```python
from build123d import *

# Parameters (mm, degrees)
F9_DEPTH      = 3.175
F9_DEPTH_BACK = 6.35
F7_R          = 3.175
F10_DEPTH     = 3.176
F3_R          = 13.0054161967
F4_R          = 1.5875
F11_DEPTH     = 6.351


# Not quite as in the source:
# - a variable given as a bare number and used for a length is read in inches; the dataset says mm whatever the document's units were


with BuildPart() as f9:
    # F1 (on Front) → F9 (new body, two sides)
    with BuildSketch(Plane.XZ) as f9_sk:
        with BuildLine():
            Line((0, 50.8), (0, 0))
            Line((0, 0), (50.8, 0))
            Line((50.8, 0), (50.8, 25.4))
            ThreePointArc((50.8, 25.4), (32.8394877579, 32.8394877579), (25.4, 50.8))
            Line((25.4, 50.8), (0, 50.8))
        make_face()
    extrude(amount=F9_DEPTH)
    extrude(f9_sk.sketch, amount=-F9_DEPTH_BACK)

    # F8 (on Front) + F7 (on Front) → F10 (cut, through all)
    with BuildSketch(Plane.XZ):
        with BuildLine():
            Line((22.8825640303, 25.1276280605), (21.4592504682, 23.7043144985))
            Line((21.4592504682, 23.7043144985), (23.7043144985, 21.4592504682))
            Line((23.7043144985, 21.4592504682), (25.1276280605, 22.8825640303))
            ThreePointArc((25.1276280605, 22.8825640303), (25.1276280605, 25.1276280605), (22.8825640303, 25.1276280605))
        make_face()
    with BuildSketch(Plane.XZ):
        with Locations((20.6375, 20.6375)):
            Circle(F7_R)
    extrude(amount=F10_DEPTH, mode=Mode.SUBTRACT)

    # F3 (on Front) + F4 (on Front) + F6 (on face) → F11 (cut, through all)
    with BuildSketch(Plane.XZ):
        with Locations((20.6375, 20.6375)):
            Circle(F3_R)
    with BuildSketch(Plane.XZ):
        with Locations((37.4589580984, 20.6375)):
            Circle(F4_R)
        with Locations((20.6375, 37.4589580984)):
            Circle(F4_R)
        with Locations((5.159375, 5.159375)):
            Circle(F4_R)
    with BuildSketch(Plane.XZ):
        Polygon((17.0707799442, 8.1307274949), (13.0054161967, 0), (28.2695838033, 0), (24.7028637475, 8.1307274949), align=None)
        Polygon((8.1307274949, 24.7028637475), (0, 28.2695838033), (0, 13.0054161967), (8.1307274949, 17.0707799442), align=None)
    extrude(amount=-F11_DEPTH, mode=Mode.SUBTRACT)


solid = f9.part
```
Could you check a few things on this model? Use its own coordinates, in mm. A direction names the side the tool comes from. Coordinates: 2 decimals unless noted, no trailing zeros. Write each loop counter-clockwise with the first axis right and the second up, starting at its lowest first coordinate (ties: lowest second). Pieces come first, ordered by that corner, then holes. Notation, with made-up numbers: (58.5, 26) -> (71.5, 26) arc R13 ccw to (71.5, 30) -> close; hole circle Ø10 at (2.25, -3.75). An arc over 180 degrees is marked (long way). Write item = value, one per line. Start each with the question number.
(1) I want a section at D-D (z = 14.5). Please give me the cut outline in (x, y) (3 decimals), plus the area to 3 significant figures.
(2) We'd pull the mould along Z, two halves only. Please class faces 4 (the face through (31, 6.35, 31)), 5 (the face through (17, 0, 17)), 6 (the face through (13, 2, 50.8)), 7 (the face through (4.01, 3.13, 15.01)): released by +Z, released by -Z, zero draft, split by the parting line, or undercut.
(3) Will these pins go through, and if not, where does the flat tip stop? pin 1 (2 mm diameter, centred on x = 23.5, y = 2.5, fed in from -Z); pin 2 (1 mm diameter, centred on x = 38, z = 20, fed in from +Y).
(4) I want a section at C-C (z = 26.5). Please give me the cut outline in (x, y) (3 decimals), plus the area to 3 significant figures.
(5) Which directions (+Z, -Z, +X, -X, +Y, -Y) give clear straight access to the entire face, cutting with the end or side of a thin tool? Please do faces 1 (the face through (4.122, 3.131, 26.461)), 2 (the face through (15.067, 3.131, 4.122)), 3 (the face through (4.82, 3.13, 3.61)).
(6) I need wall thicknesses on line 1 (Z direction, x = 20.5, y = 5.5); line 2 (Z direction, x = 5.5, y = 1.75). Which ranges of each line are inside material? Lowest first, please. Write a range as [from, to].
(7) I want a section at B-B (x = 31.5). Please give me the cut outline in (y, z) (3 decimals), plus the area to 3 significant figures.
Result set:
q1.outline = (0, -3.175) -> (50.8, -3.175) -> (50.8, 6.35) -> (32.104, 6.35) -> (32.104, 0) -> (9.171, 0) -> (9.171, 6.35) -> (2.989, 6.35) -> (2.989, 0) -> (0, 0) -> close
q1.area = 319 mm2
q2.face_4 = zero draft
q2.face_5 = undercut
q2.face_6 = released by +Z
q2.face_7 = undercut
q3.pin_1 = 8.13
q3.pin_2 = 0
q4.outline = (0, -3.175) -> (43.406, -3.175) -> (43.406, 6.35) -> (32.247, 6.35) -> (32.247, 0) -> (9.028, 0) -> (9.028, 6.35) -> (4.034, 6.35) -> (4.034, 0) -> (0, 0) -> close
q4.area = 240 mm2
q5.face_1 = -X, +Y
q5.face_2 = -Z, +Y
q5.face_3 = +Y
q6.line_1 = [33.64, 35.88], [39.04, 50.8]
q6.line_2 = [0, 3.61], [6.71, 15.76], [25.86, 50.8]
q7.outline = (-3.175, 0) -> (6.35, 0) -> (6.35, 13.486) -> (0, 13.486) -> (0, 27.789) -> (6.35, 27.789) -> (6.35, 34.287) -> (-3.175, 34.287) -> close
q7.area = 236 mm2
